Source: CAD feature listing. Evaluate the final solid. Frame: model axes, mm. A direction names the side the tool comes from. Give positions to 0.01 mm unless a question says otherwise; leave off trailing zeros. Order: outer loops, then holes, each group sorted by start corner. A loop starts at its lowest first (then second) coordinate and runs counter-clockwise, first axis right, second up. Notation, with made-up numbers: M -2.5,35.5 L 9.5,35.5 A7 ccw 9.5,45.5 Z; hole C 83,37.5 d9. An arc over 180 degrees is marked long. Answer as a JSON object with one key per item and string values. Group by question number.
1. Material intervals for L1, parallel to Y at x = 0, z = 7.75; L2, parallel to Z at x = -1.5, y = -1.5; L3, parallel to Y at x = -0.05, z = 1.25, sorted ascending. Write a range as [from, to].
2. Set-up query: faces 3 (the flat face through (0, -2, 8)), 4 (the flat face through (-0.4, -6.5, 3.3)). Return all of +Z, -Z, +X, -X, +Y, -Y with unobstructed straight access to the full face (end or side cutting, diameter ignored); none if empty.
3. Pull-direction query (Y, two-part tool) for faces 1 (the flat face through (0.4, -6.4, 2.8)), 2 (the cylindrical face through (1.717, 0.541, 7.754)); classes: +Y half, -Y half, draft (parallel to the pull), parting line (faces both ways), or undercut.
4. Section query B-B (x = 1.2). Output: boundary loops of the cut face in (y, z).
5. Section query D-D (x = -2.2). Output: boundary loops of the cut face in (y, z), plus the area to 3 significant figures.
6. Section query C-C (y = -3.5). Output: boundary loops of the cut face in (x, z).
7. Pin query (flat end, axial travel): P1, Ø0.6, axis at x = 2, z = 8, coming from the -Y side; P2, Ø3, axis at x = -1, z = 5.5, coming from the +Y side; P3, Ø2, axis at y = -5, z = 3, coming from the -X side; P4, Ø3, axis at y = -5.5, z = 2.5, coming from the +X side. Return the tip coordinate at first contact, or that it passes through.
8. Section query A-A (y = 0). Output: boundary loops of the cut face in (x, z), plus the area to 3 significant figures.
from build123d import *

# Parameters (mm, degrees)
SKETCH008_W     = 5.8
SKETCH008_H     = 6
PAD002_DEPTH    = 0.5
FILLET001_R     = 0.4
SKETCH009_W     = 1.5
SKETCH009_H     = 0.5
PAD003_DEPTH    = 1
SKETCH010_W     = 0.8
SKETCH010_H     = 0.5
FILLET002_R     = 0.35
SKETCH024_R     = 1.8
POCKET008_DEPTH = 0.5


with BuildPart() as part:
    # Sketch008 (on Face1 of CopyPocket005) → Pad002 (new body)
    with BuildSketch(Plane.XY.offset(9.5)):
        Rectangle(SKETCH008_W, SKETCH008_H)
    extrude(amount=PAD002_DEPTH)

    # Fillet001
    fillet001_edges = [part.edges().sort_by_distance(p)[0] for p in [
        (2.9, -3, 9.75),
        (-2.9, -3, 9.75),
        (-2.9, 3, 9.75),
        (2.9, 3, 9.75),
    ]]
    fillet(fillet001_edges, radius=FILLET001_R)

    # Sketch009 (on Face10 of Fillet001) → Pad003 (join)
    with BuildSketch(Plane.XZ.offset(3)):
        with Locations((0, 9.75)):
            Rectangle(SKETCH009_W, SKETCH009_H)
    extrude(amount=PAD003_DEPTH)

    # AdditivePipe: sweep along a path in Sketch011
    with BuildLine(Plane.YZ.offset(0.75)) as additivepipe_path:
        Line((-4, 9.75), (-5.434939, 9.75))
        ThreePointArc((-5.434939, 9.75), (-6.155244, 9.48897), (-6.48, 8.795061))
        Line((-6.48, 8.795061), (-6.48, -1.55))
    # Sketch010 (on Face16 of Pad003) → AdditivePipe (sweep)
    with BuildSketch(Plane.XZ.offset(4)):
        with Locations((0, 9.75)):
            Rectangle(SKETCH010_W, SKETCH010_H)
    sweep(path=additivepipe_path.line)

    # Fillet002
    fillet002_edges = [part.edges().sort_by_distance(p)[0] for p in [
        (-0.4, -6.48, -1.55),
        (0.4, -6.48, -1.55),
    ]]
    fillet(fillet002_edges, radius=FILLET002_R)

    # Sketch024 (on Face32 of Fillet002) → Pocket008 (cut)
    with BuildSketch(Plane.XY.offset(10)):
        Circle(SKETCH024_R)
    extrude(amount=-POCKET008_DEPTH, mode=Mode.SUBTRACT)


with BuildPart() as part_1:
    # Body001 placement: moved
    add(part.part.moved(Location((0, 0, -2))))


solid = part_1.part
Answer sheet:
{
 "1": {"L1": "[-6.23, -1.8], [1.8, 3]", "L2": "[7.5, 8]", "L3": "[-6.73, -6.23]"},
 "2": {"face 3": "+Z, +X, -X, +Y, -Y", "face 4": "+Z, -Z, -X, -Y"},
 "3": {"face 1": "draft", "face 2": "undercut"},
 "4": {"outline": "M -3,7.5 L -1.34,7.5 L -1.34,8 L -3,8 Z; M 1.34,7.5 L 3,7.5 L 3,8 L 1.34,8 Z"},
 "5": {"outline": "M -3,7.5 L 3,7.5 L 3,8 L -3,8 Z", "area": "3.00 mm^2"},
 "6": {"outline": "M -0.75,7.5 L 0.75,7.5 L 0.75,8 L -0.75,8 Z"},
 "7": {"P1": "y = -3", "P2": "y = -6.22", "P3": "through", "P4": "x = 0.4"},
 "8": {"outline": "M -2.9,7.5 L -1.8,7.5 L -1.8,8 L -2.9,8 Z; M 1.8,7.5 L 2.9,7.5 L 2.9,8 L 1.8,8 Z", "area": "1.10 mm^2"}
}
